from build123d import *

# Parameters (mm, degrees)
F0_W     = 11.75
F0_H     = 50
F1_DEPTH = 16
F2_R     = 1.5
F3_DEPTH = 16.001
F4_W     = 11.75
F4_H     = 9
F5_DEPTH = 10
F6_R     = 1.5
F7_DEPTH = 9.001


with BuildPart() as f1:
    # F0 (on Front) → F1 (new body)
    with BuildSketch(Plane.XZ):
        Rectangle(F0_W, F0_H)
    extrude(amount=F1_DEPTH)

    # F2 (on face) → F3 (cut, through all)
    with BuildSketch(Plane.XZ.offset(16)):
        with Locations((0, 20.2)):
            Circle(F2_R)
        with Locations((0, -10.8)):
            Circle(F2_R)
    extrude(amount=-F3_DEPTH, mode=Mode.SUBTRACT)

    # F4 (on face) → F5 (join)
    with BuildSketch(Plane.XZ.offset(16)):
        with Locations((0, -20.5)):
            Rectangle(F4_W, F4_H)
    extrude(amount=F5_DEPTH)

    # F6 (on face) → F7 (cut, through all)
    with BuildSketch(Plane.XY.offset(-16)):
        with Locations((0, -22.8)):
            Circle(F6_R)
    extrude(amount=-F7_DEPTH, mode=Mode.SUBTRACT)


solid = f1.part
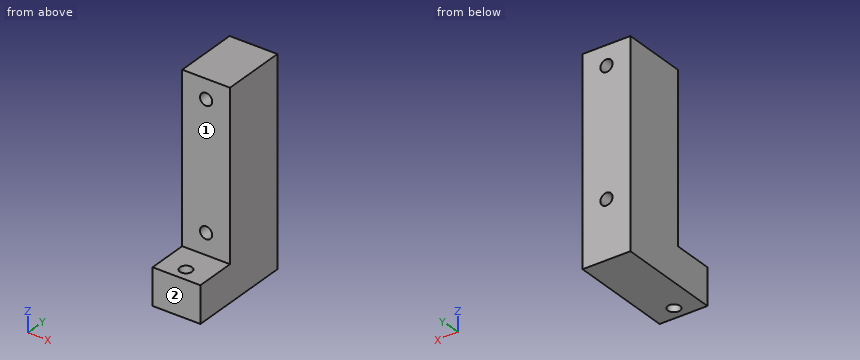
Verification items for the finished model (mm, model axes). Face numbers are marked on the shaded views. A direction names the side the tool comes from. Give positions to 0.01 mm unless a question says otherwise; leave off trailing zeros. Loops run counter-clockwise (first coordinate to the right, second up) from the corner with the lowest first, then second, coordinate; pieces in that order, holes last. Notation, with made-up numbers: (-16, 1.25) - (42, 1.25) arc R13 cw to (42, 16.25) - close; hole circle Ø5 at (75, 73.25). An arc over 180 degrees is marked (long way). Write each question's results on one line, items separated by ' | '.
1) Sectioned sample at B-B on z = 20.2. Record the boundary of the cut face in (x, y) (3 decimals).
Solution:
outline: (-5.875, -16) - (-1.5, -16) - (-1.5, 0) - (-5.875, 0) - close; (1.5, -16) - (5.875, -16) - (5.875, 0) - (1.5, 0) - close
2) Depth check by flat-ended pin: P1, Ø2.5, axis at x = 0, z = -10.8, coming from the -Y side; P2, Ø5, axis at x = 2, z = 9, coming from the +Y side; P3, Ø4, axis at x = 0, y = -22.8, coming from the +Z side; P4, Ø1, axis at x = -3, z = -10.5, coming from the -Y side. Enter the tip coordinate at first touch or a pass-through.
Solution:
P1: through | P2: y = 0 | P3: z = -16 | P4: y = -16
3) Sectioned sample at D-D on z = -18. Record the boundary of the cut face in (x, y) (3 decimals), plus the area to 3 significant figures.
Solution:
outline: (-5.875, -26) - (5.875, -26) - (5.875, 0) - (-5.875, 0) - close; hole circle Ø3 at (0, -22.8) | area: 298 mm2
4) Sectioned sample at C-C on x = 0. Record the boundary of the cut face in (y, z).
Solution:
outline: (-26, -25) - (-24.3, -25) - (-24.3, -16) - (-26, -16) - close; (-21.3, -25) - (0, -25) - (0, -12.3) - (-16, -12.3) - (-16, -16) - (-21.3, -16) - close; (-16, -9.3) - (0, -9.3) - (0, 18.7) - (-16, 18.7) - close; (-16, 21.7) - (0, 21.7) - (0, 25) - (-16, 25) - close
5) Tool access check on the marked faces 1 and 2. Record the directions out of +Z, -Z, +X, -X, +Y, -Y that give a thin tool (end or side, any length) a straight path to the whole face; none if there is none.
Solution:
face 1: +Z, +X, -X, -Y | face 2: +Z, -Z, +X, -X, -Y
6) Sectioned sample at A-A on y = -22.8. Record the boundary of the cut face in (x, z) (3 decimals), plus the area to 4 significant figures.
Solution:
outline: (-5.875, -25) - (-1.5, -25) - (-1.5, -16) - (-5.875, -16) - close; (1.5, -25) - (5.875, -25) - (5.875, -16) - (1.5, -16) - close | area: 78.75 mm2
7) Material ranges on L1, parallel to Z at x = 0, y = -6; L2, parallel to Y at x = 0, z = -20.25; L3, parallel to Y at x = -1.5, z = -6.5, recorded low to high. Write a range as from..to.
Solution:
L1: -25..-12.3, -9.3..18.7, 21.7..25 | L2: -26..-24.3, -21.3..0 | L3: -16..0
